The listing builds one solid part. Answer for the finished solid, in the listing's coordinates (mm). A direction names the side the tool comes from. Give positions to 0.01 mm unless a question says otherwise; leave off trailing zeros. Write each loop counter-clockwise with the first axis right and the second up, starting at its lowest first coordinate (ties: lowest second). Pieces come first, ordered by that corner, then holes. Notation, with made-up numbers: (-35, 82.25) -> (-5, 82.25) arc R26 ccw to (-5, 112.25) -> close; hole circle Ø3 at (81, -27). An arc over 180 degrees is marked (long way). Put each result on its own line as item: value. Start each with the question number.
1) For faces 1 (the flat face through (-1, -28.75, 39)), 2 (the flat face through (-1, -31, 10)), 3 (the flat face through (-40, 0, 30)), 4 (the flat face through (40, 0, 30)), 5 (the flat face through (4.79, 31.831, 67.005)), determine the directions among +Z, -Z, +X, -X, +Y, -Y from which every point of the face is accessible in a straight line to the end or side of a thin tool.
2) A cutting plane is placed at B-B (z = 30). Write down the section's boundary in (x, y), then the cut area to 3 significant figures.
3) Flat-ended cylindrical pins translate along their axes: pin 1 Ø6 at (x, y) = (39.5, -9) entering from +Z; pin 2 Ø12 at (y, z) = (-9, 37) entering from +X; pin 3 Ø5 at (y, z) = (13.5, 3.5) entering from -X. Find the tip coordinate at first contact, or state that the pin passes through.
4) Find the intervals of material crossed by line 1 along Z through (x, y) = (25, 32); line 2 along Y through (x, z) = (6.5, 40); line 3 along Y through (x, z) = (42.5, 51), in increasing order. Write a range as from..to.
5) For a pull along Z with two mould halves and no side action, classify faces 6 (the flat face through (7.48, -0.49, 79)), 7 (the flat face through (4.79, -31.919, 67.005)), 8 (the flat face through (-52.5, 0, 5)), 9 (the flat face through (22, -18.75, 30)) as released by +Z, released by -Z, zero draft, split by the parting line, or undercut.
6) A cutting plane is placed at C-C (y = -17). Write down the section's boundary in (x, z).
7) A cutting plane is placed at A-A (y = -33). Write down the section's boundary in (x, z), then the cut area to 3 significant figures.
8) A cutting plane is placed at D-D (x = -17). Write down the section's boundary in (y, z), then the cut area to 3 significant figures.
from build123d import *

# Parameters (mm, degrees)
F0_W      = 105
F0_H      = 70
F1_DEPTH  = 10
F2_W      = 80
F2_H      = 57.5
F3_DEPTH  = 40
F5_DEPTH  = 57.5
F7_DEPTH  = 70
F8_R      = 2.5
F9_DEPTH  = 10
F10_R     = 10
F11_DEPTH = 10
F12_R     = 10
F13_DEPTH = 10


with BuildPart() as f1:
    # F0 (on Top) → F1 (new body)
    with BuildSketch(Plane.XY):
        Rectangle(F0_W, F0_H)
    extrude(amount=F1_DEPTH)

    # F2 (on face) → F3 (join)
    with BuildSketch(Plane.XY.offset(10)):
        Rectangle(F2_W, F2_H)
    extrude(amount=F3_DEPTH)

    # F4 (on face) → F5 (join)
    with BuildSketch(Plane.XZ.offset(28.75)):
        Polygon((-10, 83.54102), (-40, 50), (20, 50), align=None)
    extrude(amount=-F5_DEPTH)

    # F6 (on face) → F7 (join, through all)
    with BuildSketch(Plane.XZ.offset(35)):
        Polygon((20, 50), (45, 50), (45, 60), (24.472136, 60), (-10, 98.54102), (-54.120227, 49.213107), (-46.666667, 42.54644), (-40, 50), (-10, 83.54102), align=None)
    extrude(amount=-F7_DEPTH)

    # F8 (on face) → F9 (join)
    with BuildSketch(Plane.XZ.offset(28.75)):
        with Locations((-10, 37.5)):
            Circle(F8_R)
    extrude(amount=F9_DEPTH)

    # F10 (on face) → F11 (cut)
    with BuildSketch(Plane.XZ.offset(28.75)):
        with Locations((22.5, 30)):
            Circle(F10_R)
    extrude(amount=-F11_DEPTH, mode=Mode.SUBTRACT)

    # F12 (on face) → F13 (cut)
    with BuildSketch(Plane.XZ.offset(28.75)):
        with Locations((-10, 60)):
            Circle(F12_R)
    extrude(amount=-F13_DEPTH, mode=Mode.SUBTRACT)


solid = f1.part
Reply:
1. face 1: -Y
1. face 2: none
1. face 3: +Y, -Y
1. face 4: +X, +Y, -Y
1. face 5: +Y
2. outline: (-40, -28.75) -> (12.5, -28.75) -> (12.5, -18.75) -> (32.5, -18.75) -> (32.5, -28.75) -> (40, -28.75) -> (40, 28.75) -> (-40, 28.75) -> close
2. area: 4,400 mm2
3. pin 1: stops at z = 60
3. pin 2: stops at x = 40
3. pin 3: stops at x = -52.5
4. line 1: z = 0..10, 50..60
4. line 2: y = -28.75..28.75
4. line 3: y = -35..35
5. face 6: released by +Z
5. face 7: undercut
5. face 8: zero draft
5. face 9: undercut
6. outline: (-54.12, 49.21) -> (-46.67, 42.55) -> (-40, 50) -> (-40, 10) -> (-52.5, 10) -> (-52.5, 0) -> (52.5, 0) -> (52.5, 10) -> (40, 10) -> (40, 50) -> (45, 50) -> (45, 60) -> (24.47, 60) -> (-10, 98.54) -> close
7. outline: (-54.12, 49.21) -> (-46.67, 42.55) -> (-10, 83.54) -> (20, 50) -> (45, 50) -> (45, 60) -> (24.47, 60) -> (-10, 98.54) -> close; (-52.5, 0) -> (52.5, 0) -> (52.5, 10) -> (-52.5, 10) -> close; circle Ø5 at (-10, 37.5)
7. area: 2,390 mm2
8. outline: (-35, 0) -> (35, 0) -> (35, 10) -> (28.75, 10) -> (28.75, 75.71) -> (35, 75.71) -> (35, 90.71) -> (-35, 90.71) -> (-35, 75.71) -> (-28.75, 75.71) -> (-28.75, 67.14) -> (-18.75, 67.14) -> (-18.75, 52.86) -> (-28.75, 52.86) -> (-28.75, 10) -> (-35, 10) -> close
8. area: 5,390 mm2
